Build history of the part. All positions in model axes, mm. A direction names the side the tool comes from. Coordinates: 2 decimals unless noted, no trailing zeros. Order: outer loops, then holes, each group sorted by start corner. A loop starts at its lowest first (then second) coordinate and runs counter-clockwise, first axis right, second up. Notation, with made-up numbers: M 77.25,56.25 L 108.25,56.25 A18 ccw 108.25,89.25 Z; hole C -25.75,17 d2. An arc over 180 degrees is marked long. Use a Markdown table: item, result. Add a question column.
from build123d import *

# Parameters (mm, degrees)
SALIENTE_EXTRUIR1_DEPTH = 100
CROQUIS3_R              = 5
CROQUIS3_R_2            = 3.5
CROQUIS3_W              = 52.452137676
CROQUIS3_H              = 23.4
CORTAR_EXTRUIR1_DEPTH   = 2
CORTAR_EXTRUIR2_REACH   = 107.333
CROQUIS4_W              = 27.547862324
CROQUIS4_H              = 23.4


with BuildPart() as part:
    # Croquis2 → Saliente-Extruir1 (new body)
    with BuildSketch(Plane(origin=(0, 0, 0), x_dir=(0, 0, -1), z_dir=(1, 0, 0))):
        Polygon((0, 0), (-21.4, 0), (-21.4, -21.4), (-21.4, -23.4), (-23.4, -23.4), (-23.4, 2), (2, 2), (2, 0), align=None)
    extrude(amount=SALIENTE_EXTRUIR1_DEPTH)

    # Croquis3 → Cortar-Extruir1 (cut)
    with BuildSketch(Plane(origin=(0, 2, 0), x_dir=(1, 0, 0), z_dir=(0, 1, 0))):
        with Locations(Location((7, -4.7, 0), (0, 0, 270))):
            Circle(CROQUIS3_R)
        with Locations(Location((22, -4.7, 0), (0, 0, 270))):
            Circle(CROQUIS3_R_2)
        with Locations((73.773931162, -9.7)):
            Rectangle(CROQUIS3_W, CROQUIS3_H)
        Polygon((0, -21.4), (0, -11.4), (27.547862324, -11.4), (27.547862324, -21.4), (27.547862324, -23.4), (0, -23.4), align=None)
    extrude(amount=-CORTAR_EXTRUIR1_DEPTH, mode=Mode.SUBTRACT)

    # Croquis4 → Cortar-Extruir2 (cut, up to next)
    with BuildSketch(Plane(origin=(0, 0, 21.4), x_dir=(-1, 0, 0), z_dir=(0, 0, -1)), mode=Mode.PRIVATE) as cortar_extruir2_sk1:
        with Locations((-13.773931162, -11.7)):
            Rectangle(CROQUIS4_W, CROQUIS4_H)
    cortar_extruir2_tool1 = extrude(cortar_extruir2_sk1.sketch, amount=-CORTAR_EXTRUIR2_REACH, mode=Mode.PRIVATE) & part.part
    add(cortar_extruir2_tool1.solids().sort_by_distance((13.773931, -11.7, 21.4))[0], mode=Mode.SUBTRACT)


solid = part.part
(1) Mould opens along Z. For faces 5 (the cylindrical face through (8.5, 1.01, 9.47)), 6 (the cylindrical face through (25.47, 1.01, 4.24)), 7 (the flat face through (39, 2, 10)), 8 (the flat face through (23, 1, -2)) say: released by +Z, released by -Z, zero draft, split by the parting line, or undercut.
(2) Slice it at C-C on x = 7. Give the cut face in (y, z), and give its area (3 significant figures).
(3) Drill centre lines: line 1 along X through (y, z) = (0.5, 4.7); line 2 along X through (y, z) = (0.5, 6.5); line 3 along Z through (x, y) = (49, -3.75). Where is each one in solid material? Low to high. Write a range as from..to.
(4) Slice it at A-A on x = 22. Give the cut face in (y, z).
(5) Slice it at D-D on y = -7.75. Give the cut face in (x, z), and give its area (3 significant figures).
(6) Slice it at B-B on z = 4.7. Give the cut face in (x, y).
(7) Drop flat-ended pins along their axis: P1, Ø1, axis at x = 15, z = 1, coming from the -Y side; P2, Ø12, axis at y = -11, z = 20.5, coming from the -X side; P3, Ø2, axis at x = 9, y = 1, coming from the +Z side. Give the stop position or say it passes through.
(8) Which spindle directions (+Z, -Z, +X, -X, +Y, -Y) get a long thin tool onto all of the face, cutting with end or side? Do faces 1 (the flat face through (14, 1, 11.4)), 2 (the flat face through (29, 0, 7)), 3 (the flat face through (47.548, 1, 10)), 4 (the flat face through (63, -23.4, 22)). Say none if no direction does.
Solutions:
| question | item | result |
|---|---|---|
| 1 | face 5 | undercut |
| 1 | face 6 | undercut |
| 1 | face 7 | zero draft |
| 1 | face 8 | released by -Z |
| 2 | outline | M 0,-2 L 2,-2 L 2,-0.3 L 0,-0.3 Z; M 0,9.7 L 2,9.7 L 2,11.4 L 0,11.4 Z |
| 2 | area | 6.80 mm² |
| 3 | line 1 | 0..2, 12..18.5, 25.5..47.55 |
| 3 | line 2 | 0..2.34, 11.66..19, 25..47.55 |
| 3 | line 3 | 21.4..23.4 |
| 4 | outline | M 0,-2 L 2,-2 L 2,1.2 L 0,1.2 Z; M 0,8.2 L 2,8.2 L 2,11.4 L 0,11.4 Z |
| 5 | outline | M 27.55,21.4 L 100,21.4 L 100,23.4 L 27.55,23.4 Z |
| 5 | area | 145 mm² |
| 6 | outline | M 0,0 L 2,0 L 2,2 L 0,2 Z; M 12,0 L 18.5,0 L 18.5,2 L 12,2 Z; M 25.5,0 L 47.55,0 L 47.55,2 L 25.5,2 Z |
| 7 | P1 | y = 0 |
| 7 | P2 | x = 27.55 |
| 7 | P3 | z = 11.4 |
| 8 | face 1 | +Z, -X, +Y, -Y |
| 8 | face 2 | -Z, +X, -X, -Y |
| 8 | face 3 | -Z, +X, +Y, -Y |
| 8 | face 4 | +Z, -Z, +X, -X, -Y |
